The listing builds one solid part. Answer for the finished solid, in the listing's coordinates (mm). Face numbers are marked on the shaded views. Coordinates: 2 decimals unless noted, no trailing zeros. Write each loop counter-clockwise with the first axis right and the second up, starting at its lowest first coordinate (ties: lowest second). Pieces come first, ordered by that corner, then holes.
from build123d import *

# Parameters (mm, degrees)
PIPE_TAP_DRILL_FOR_1_4_TAP1_D = 11.1252
PIPE_TAP_DRILL_FOR_1_8_TAP1_D = 8.4328
SKETCH6_R                     = 6.35
BOSS_EXTRUDE1_DEPTH           = 6.35


with BuildPart() as part:
    # Sketch1 → Revolve1 (revolve)
    with BuildSketch(Plane.XY, mode=Mode.PRIVATE) as revolve1_sk:
        Polygon((0, 0), (47.498, 0), (47.498, 2.4638), (44.577, 2.4638), (44.577, 7.4422), (47.498, 7.4422), (47.498, 9.906), (41.148, 9.906), (41.148, 6.35), (0, 6.35), align=None)
    revolve(revolve1_sk.sketch.rotate(Axis((0, 48.192213231, 0), (0, -1, 0)), 180), axis=Axis((0, 48.192213231, 0), (0, -1, 0)))

    # Pipe Tap Drill for 1/4 Tap1 (through all)
    with Locations(Plane(origin=(0, 6.35, 0), x_dir=(1, 0, 0), z_dir=(0, 1, 0))):
        with Locations((0, 0), (-30.1752, 0)):
            Hole(PIPE_TAP_DRILL_FOR_1_4_TAP1_D / 2)

    # Pipe Tap Drill for 1/8 Tap1 (through all)
    with Locations(Plane(origin=(0, 6.35, 0), x_dir=(1, 0, 0), z_dir=(0, 1, 0))):
        with Locations((12.150198978, -29.333175157)):
            Hole(PIPE_TAP_DRILL_FOR_1_8_TAP1_D / 2)

    # Sketch6 → Boss-Extrude1 (add)
    with BuildSketch(Plane(origin=(0, 6.35, 0), x_dir=(1, 0, 0), z_dir=(0, 1, 0))):
        Circle(SKETCH6_R)
    extrude(amount=-BOSS_EXTRUDE1_DEPTH)


solid = part.part
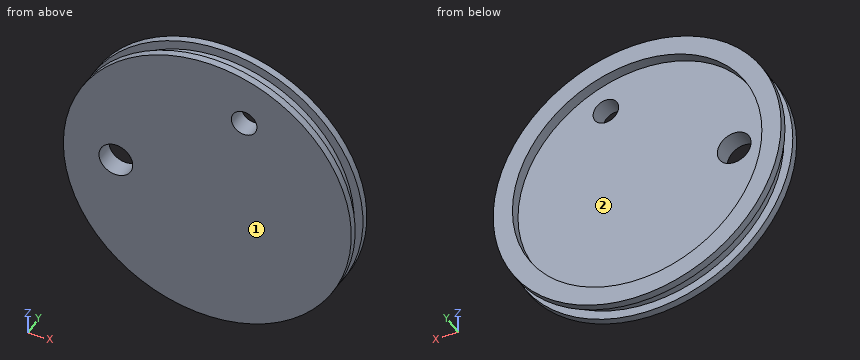
1. For a pull along X with two mould halves and no side action, classify the marked faces 1 and 2 as pulls with the +X half, pulls with the -X half, needs draft (parallel to the pull), parting line crosses it, or undercut.
Results found:
face 1: needs draft
face 2: undercut
2. Section B-B on x = 12 is taken. Give the vertices of the cut face in (y, z), then the cut area to 3 significant figures.
Results found:
outline: (0, -45.96) - (2.46, -45.96) - (2.46, -42.93) - (7.44, -42.93) - (7.44, -45.96) - (9.91, -45.96) - (9.91, -39.36) - (6.35, -39.36) - (6.35, 25.12) - (0, 25.12) - close; (0, 33.55) - (6.35, 33.55) - (6.35, 39.36) - (9.91, 39.36) - (9.91, 45.96) - (7.44, 45.96) - (7.44, 42.93) - (2.46, 42.93) - (2.46, 45.96) - (0, 45.96) - close
area: 547 mm2
3. Find the intervals of material crossed by L1, parallel to Z at x = 0, y = 7.5; L2, parallel to Z at x = -21, y = 9; L3, parallel to Y at x = 12.5, z = 3.5, in increasing order.
Results found:
L1: z = -47.5 to -41.15, 41.15 to 47.5
L2: z = -42.6 to -35.39, 35.39 to 42.6
L3: y = 0 to 6.35
4. Section A-A on z = 0 is taken. Give the vertices of the cut face in (x, y), then the cut area to 3 significant figures.
Results found:
outline: (-47.5, 0) - (-35.74, 0) - (-35.74, 6.35) - (-41.15, 6.35) - (-41.15, 9.91) - (-47.5, 9.91) - (-47.5, 7.44) - (-44.58, 7.44) - (-44.58, 2.46) - (-47.5, 2.46) - close; (-24.61, 0) - (47.5, 0) - (47.5, 2.46) - (44.58, 2.46) - (44.58, 7.44) - (47.5, 7.44) - (47.5, 9.91) - (41.15, 9.91) - (41.15, 6.35) - (-24.61, 6.35) - close
area: 549 mm2
5. Flat-ended cylindrical pins translate along their axes: P1, Ø1, axis at y = 2, z = -5, coming from the +X side; P2, Ø1, axis at x = -6, z = -4.5, coming from the +Y side; P3, Ø24.5, axis at x = 10.5, z = -20.5, coming from the +Y side. Find the tip coordinate at first contact, or state that the pin passes through.
Results found:
P1: stops at x = 47.28
P2: stops at y = 6.35
P3: stops at y = 6.35
6. Section D-D on z = -40 is taken. Give the vertices of the cut face in (x, y).
Results found:
outline: (-25.61, 0) - (25.61, 0) - (25.61, 2.46) - (19.68, 2.46) - (19.68, 7.44) - (25.61, 7.44) - (25.61, 9.91) - (9.65, 9.91) - (9.65, 6.35) - (-9.65, 6.35) - (-9.65, 9.91) - (-25.61, 9.91) - (-25.61, 7.44) - (-19.68, 7.44) - (-19.68, 2.46) - (-25.61, 2.46) - close
7. Section C-C on x = 0 is taken. Give the vertices of the cut face in (y, z), then the cut area to 3 significant figures.
Results found:
outline: (0, -47.5) - (2.46, -47.5) - (2.46, -44.58) - (7.44, -44.58) - (7.44, -47.5) - (9.91, -47.5) - (9.91, -41.15) - (6.35, -41.15) - (6.35, 41.15) - (9.91, 41.15) - (9.91, 47.5) - (7.44, 47.5) - (7.44, 44.58) - (2.46, 44.58) - (2.46, 47.5) - (0, 47.5) - close
area: 619 mm2
